Work out the finished part from the listing and answer in its coordinate system (mm). Face numbers are marked on the shaded views. A direction names the side the tool comes from. Coordinates: 2 decimals unless noted, no trailing zeros. Order: outer loops, then holes, each group sorted by start corner. A loop starts at its lowest first (then second) coordinate and runs counter-clockwise, first axis right, second up. Notation, with made-up numbers: M 25,34.25 L 73,34.25 A21 cw 73,56.25 Z; hole C 36.5,-28.75 d3. An arc over 180 degrees is marked long. Use a Markdown table: item, result.
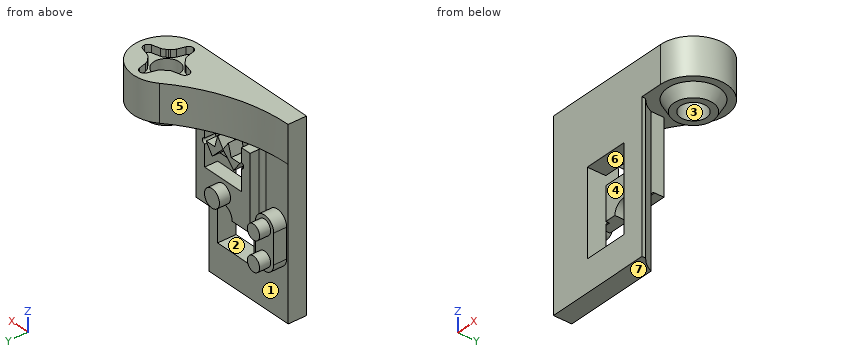
from build123d import *

# Parameters (mm, degrees)
SKETCH2_R           = 9
BOSS_EXTRUDE1_DEPTH = 10
SKETCH3_R           = 7
BOSS_EXTRUDE2_DEPTH = 3
BOSS_EXTRUDE2_TAPER = 30
CUT_EXTRUDE1_DEPTH  = 2
BOSS_EXTRUDE3_DEPTH = 40
SKETCH6_W           = 12
SKETCH6_H           = 23
CUT_EXTRUDE3_DEPTH  = 55.717456081
BOSS_EXTRUDE4_DEPTH = 3.5
SKETCH8_R           = 2
BOSS_EXTRUDE5_DEPTH = 3
SKETCH9_R           = 3.5
CUT_EXTRUDE4_DEPTH  = 52.720402164
BOSS_EXTRUDE6_DEPTH = 3.5
SKETCH11_R          = 2.45
BOSS_EXTRUDE7_DEPTH = 3
BOSS_EXTRUDE9_DEPTH = 3.5
FILLET1_START       = -26.74
FILLET1_DEPTH       = 2.84
FILLET1_START_2     = -11.9
FILLET1_2_DEPTH     = 2.83
FILLET1_START_3     = -21
FILLET1_3_DEPTH     = 21
FILLET1_START_4     = -27.74
FILLET1_4_DEPTH     = 1


with BuildPart() as part:
    # Sketch2 → Boss-Extrude1 (new body)
    with BuildSketch(Plane.XY):
        with BuildLine():
            Line((-35, -9), (0, -9))
            ThreePointArc((0, -9), (-8.437416666, -3.132091953), (-5.872614409, 6.82))
            ThreePointArc((-5.872614409, 6.82), (-19.465199243, -1.204217751), (-35, -4))
            Line((-35, -4), (-35, -9))
        make_face()
        Circle(SKETCH2_R)
    extrude(amount=BOSS_EXTRUDE1_DEPTH)

    # Sketch3 → Boss-Extrude2 (add)
    with BuildSketch(Plane(origin=(0, 0, 0), x_dir=(-1, 0, 0), z_dir=(0, 0, -1))):
        Circle(SKETCH3_R)
    extrude(amount=BOSS_EXTRUDE2_DEPTH, taper=BOSS_EXTRUDE2_TAPER)

    # Sketch4 → Cut-Extrude1 (cut)
    with BuildSketch(Plane.XY.offset(10)):
        with BuildLine():
            Line((1.2, -6.33), (1.8, -4.1378116))
            ThreePointArc((1.8, -4.1378116), (2.058560194, -3.569045514), (2.48, -3.1078116))
            ThreePointArc((2.48, -3.1078116), (2.64989874, -2.964295475), (2.811558399, -2.811558399))
            ThreePointArc((2.811558399, -2.811558399), (2.964295475, -2.64989874), (3.1078116, -2.48))
            ThreePointArc((3.1078116, -2.48), (3.569045514, -2.058560194), (4.1378116, -1.8))
            Line((4.1378116, -1.8), (6.33, -1.2))
            ThreePointArc((6.33, -1.2), (6.992020752, -0.754882576), (7.25, 0))
            ThreePointArc((7.25, 0), (6.992020752, 0.754882576), (6.33, 1.2))
            Line((6.33, 1.2), (4.1378116, 1.8))
            ThreePointArc((4.1378116, 1.8), (3.569045514, 2.058560194), (3.1078116, 2.48))
            ThreePointArc((3.1078116, 2.48), (2.964295475, 2.64989874), (2.811558399, 2.811558399))
            ThreePointArc((2.811558399, 2.811558399), (2.64989874, 2.964295475), (2.48, 3.1078116))
            ThreePointArc((2.48, 3.1078116), (2.058560194, 3.569045514), (1.8, 4.1378116))
            Line((1.8, 4.1378116), (1.2, 6.33))
            ThreePointArc((1.2, 6.33), (0.754882576, 6.992020752), (0, 7.25))
            ThreePointArc((0, 7.25), (-0.754882576, 6.992020752), (-1.2, 6.33))
            Line((-1.2, 6.33), (-1.8, 4.1378116))
            ThreePointArc((-1.8, 4.1378116), (-2.058560194, 3.569045514), (-2.48, 3.1078116))
            ThreePointArc((-2.48, 3.1078116), (-2.64989874, 2.964295475), (-2.811558399, 2.811558399))
            ThreePointArc((-2.811558399, 2.811558399), (-2.964295475, 2.64989874), (-3.1078116, 2.48))
            ThreePointArc((-3.1078116, 2.48), (-3.569045514, 2.058560194), (-4.1378116, 1.8))
            Line((-4.1378116, 1.8), (-6.33, 1.2))
            ThreePointArc((-6.33, 1.2), (-6.992020752, 0.754882576), (-7.25, 0))
            ThreePointArc((-7.25, 0), (-6.992020752, -0.754882576), (-6.33, -1.2))
            Line((-6.33, -1.2), (-4.1378116, -1.8))
            ThreePointArc((-4.1378116, -1.8), (-3.569045514, -2.058560194), (-3.1078116, -2.48))
            ThreePointArc((-3.1078116, -2.48), (-2.964295475, -2.64989874), (-2.811558399, -2.811558399))
            ThreePointArc((-2.811558399, -2.811558399), (-2.64989874, -2.964295475), (-2.48, -3.1078116))
            ThreePointArc((-2.48, -3.1078116), (-2.058560194, -3.569045514), (-1.8, -4.1378116))
            Line((-1.8, -4.1378116), (-1.2, -6.33))
            ThreePointArc((-1.2, -6.33), (-0.754882576, -6.992020752), (0, -7.25))
            ThreePointArc((0, -7.25), (0.754882576, -6.992020752), (1.2, -6.33))
        make_face()
    extrude(amount=-CUT_EXTRUDE1_DEPTH, mode=Mode.SUBTRACT)

    # Sketch5 → Boss-Extrude3 (add)
    with BuildSketch(Plane(origin=(0, 0, 0), x_dir=(-1, 0, 0), z_dir=(0, 0, -1))):
        with BuildLine():
            Line((35, -9), (35, -4))
            Line((35, -4), (9.07, -4))
            ThreePointArc((9.07, -4), (7.791254425, -6.196675271), (6, -8))
            Line((6, -8), (6, -9))
            Line((6, -9), (35, -9))
        make_face()
    extrude(amount=BOSS_EXTRUDE3_DEPTH)

    # Sketch6 → Cut-Extrude3 (cut, through all)
    with BuildSketch(Plane(origin=(0, -4, 0), x_dir=(1, 0, 0), z_dir=(0, 1, 0))):
        with Locations((-17.9, 20)):
            Rectangle(SKETCH6_W, SKETCH6_H)
    extrude(amount=-CUT_EXTRUDE3_DEPTH, mode=Mode.SUBTRACT)

    # Sketch7 → Boss-Extrude4 (add)
    with BuildSketch(Plane(origin=(0, -4, 0), x_dir=(1, 0, 0), z_dir=(0, 1, 0))):
        with BuildLine():
            Line((-34.5, 16), (-34.5, 24))
            ThreePointArc((-34.5, 24), (-31.5, 27), (-28.5, 24))
            Line((-28.5, 24), (-28.5, 16))
            ThreePointArc((-28.5, 16), (-31.5, 13), (-34.5, 16))
        make_face()
    extrude(amount=BOSS_EXTRUDE4_DEPTH)

    # Sketch8 → Boss-Extrude5 (add)
    with BuildSketch(Plane(origin=(0, -0.5, 0), x_dir=(1, 0, 0), z_dir=(0, 1, 0))):
        with Locations(Location((-31.5, 24, 0), (0, 0, 180))):
            Circle(SKETCH8_R)
        with Locations((-31.5, 16)):
            Circle(SKETCH8_R)
    extrude(amount=BOSS_EXTRUDE5_DEPTH)

    # Sketch9 → Cut-Extrude4 (cut, through all)
    with BuildSketch(Plane(origin=(0, 0, -3), x_dir=(-1, 0, 0), z_dir=(0, 0, -1))):
        Circle(SKETCH9_R)
    extrude(amount=-CUT_EXTRUDE4_DEPTH, mode=Mode.SUBTRACT)

    # Sketch10 → Boss-Extrude6 (add)
    with BuildSketch(Plane(origin=(0, -4, 0), x_dir=(1, 0, 0), z_dir=(0, 1, 0))):
        with BuildLine():
            Line((-26.74, 0), (-26.74, 20))
            Line((-26.74, 20), (-20.91, 20))
            ThreePointArc((-20.91, 20), (-17.91, 17), (-14.91, 20))
            Line((-14.91, 20), (-9.07, 20))
            Line((-9.07, 20), (-9.07, 0))
            Line((-9.07, 0), (-11.9, 0))
            Line((-11.9, 0), (-11.9, 3.75))
            ThreePointArc((-11.9, 3.75), (-11.15, 4.5), (-11.9, 5.25))
            Line((-11.9, 5.25), (-11.9, 11))
            Line((-11.9, 11), (-23.9, 11))
            Line((-23.9, 11), (-23.9, 5.25))
            ThreePointArc((-23.9, 5.25), (-24.65, 4.5), (-23.9, 3.75))
            Line((-23.9, 3.75), (-23.9, 0))
            Line((-23.9, 0), (-26.74, 0))
        make_face()
    extrude(amount=BOSS_EXTRUDE6_DEPTH)

    # Sketch11 → Boss-Extrude7 (add)
    with BuildSketch(Plane(origin=(0, -0.5, 0), x_dir=(1, 0, 0), z_dir=(0, 1, 0))):
        with Locations(Location((-17.905833333, 14.5, 0), (0, 0, 180))):
            Circle(SKETCH11_R)
    extrude(amount=BOSS_EXTRUDE7_DEPTH)

    # Sketch12 → Boss-Extrude9 (add)
    with BuildSketch(Plane(origin=(0, -4, 0), x_dir=(1, 0, 0), z_dir=(0, 1, 0))):
        Polygon((-20.58, 4.2), (-19.65, 1), (-17.93, 3.45), (-17.87, 3.45), (-16.15, 1), (-15.22, 4.2), (-12.4, 4.2), (-14.4, 7), (-17.85, 3.55), (-17.95, 3.55), (-21.4, 7), (-23.4, 4.2), align=None)
    extrude(amount=BOSS_EXTRUDE9_DEPTH)

    # Fillet1: read off the stored shape, not the designer's step
    # Fillet1 outline → Fillet1 (add)
    with BuildSketch(Plane.YZ.offset(FILLET1_START)):
        with BuildLine():
            ThreePointArc((-4, -21), (-3.707106781, -20.292893219), (-3, -20))
            Line((-3, -20), (-4, -20))
            Line((-4, -20), (-4, -21))
        make_face()
    extrude(amount=FILLET1_DEPTH)

    # Fillet1 2 outline → Fillet1 2 (add)
    with BuildSketch(Plane.YZ.offset(FILLET1_START_2)):
        with BuildLine():
            ThreePointArc((-4, -21), (-3.707106781, -20.292893219), (-3, -20))
            Line((-3, -20), (-4, -20))
            Line((-4, -20), (-4, -21))
        make_face()
    extrude(amount=FILLET1_2_DEPTH)

    # Fillet1 3 outline → Fillet1 3 (add)
    with BuildSketch(Plane.XY.offset(FILLET1_START_3)):
        with BuildLine():
            Line((-26.74, -4), (-26.74, -3))
            ThreePointArc((-26.74, -3), (-27.032893219, -3.707106781), (-27.74, -4))
            Line((-27.74, -4), (-26.74, -4))
        make_face()
    extrude(amount=FILLET1_3_DEPTH)

    # Fillet1 4 outline → Fillet1 4 (cut)
    with BuildSketch(Plane.YZ.offset(FILLET1_START_4)):
        with BuildLine():
            Line((-2, -19.999999999), (-3, -20))
            ThreePointArc((-3, -20), (-3.707106781, -20.292893219), (-4, -21))
            Line((-4, -21), (-2, -21))
            Line((-2, -21), (-2, -19.999999999))
        make_face()
    extrude(amount=FILLET1_4_DEPTH, mode=Mode.SUBTRACT)


solid = part.part
1. Flat-ended cylindrical pins translate along their axes: P1, Ø5.5, axis at x = -19, z = -13.5, coming from the +Y side; P2, Ø1.5, axis at x = -22, y = 3, coming from the +Z side; P3, Ø3, axis at y = -1.5, z = -7, coming from the -X side; P4, Ø6.5, axis at x = -20.5, z = -3.5, coming from the +Y side. Find the tip coordinate at first contact, or state that the pin passes through.
Answers below:
| item | result |
|---|---|
| P1 | y = 2.5 |
| P2 | through |
| P3 | x = -26.74 |
| P4 | y = -0.5 |
2. Find the intervals of material crossed by probe 1 along Z at (x, y) = (-9.5, 2.5); probe 2 along Z at (x, y) = (-4.5, 1.25); probe 3 along Y at (x, z) = (0, 2), in increasing order.
Answers below:
| item | result |
|---|---|
| probe 1 | 0 to 10 |
| probe 2 | -3 to 8 |
| probe 3 | -9 to -3.5, 3.5 to 9 |
3. Section B-B on z = -32.5 is taken. Determine the outline of the cut face in (x, y), then the cut area to 3 significant figures.
Answers below:
| item | result |
|---|---|
| outline | M -35,-9 L -6,-9 L -6,-8 A10 cw -9.07,-4 L -35,-4 Z |
| area | 138 mm² |
4. For the marked faces 5, 6 and 7, determine the directions among +Z, -Z, +X, -X, +Y, -Y from which every point of the face is accessible in a straight line to the end or side of a thin tool.
Answers below:
| item | result |
|---|---|
| face 5 | +Z, -X, +Y |
| face 6 | +Y, -Y |
| face 7 | -Z, +X, -X, +Y, -Y |
5. For a pull along Y with two mould halves and no side action, classify the marked faces 1, 2, 3 and 4 as +Y half, -Y half, draft (parallel to the pull), parting line (faces both ways), or undercut.
Answers below:
| item | result |
|---|---|
| face 1 | +Y half |
| face 2 | draft |
| face 3 | undercut |
| face 4 | -Y half |
6. Section A-A on x = -22.5 is taken. Determine the outline of the cut face in (y, z).
Answers below:
| item | result |
|---|---|
| outline | M -9,-40 L -4,-40 L -4,-31.5 L -9,-31.5 Z; M -9,-8.5 L -4,-8.5 L -4,-5.46 L -0.5,-5.46 L -0.5,-4.2 L -4,-4.2 L -4,0 L -2.21,0 L -2.21,10 L -9,10 Z; M -4,-20 L -0.5,-20 L -0.5,-11 L -4,-11 Z |
7. Section C-C on x = -8.5 is taken. Determine the outline of the cut face in (y, z), then the cut area to 3 significant figures.
Answers below:
| item | result |
|---|---|
| outline | M -9,-40 L -5.14,-40 L -5.14,0 L 4.72,0 L 4.72,10 L -9,10 Z |
| area | 292 mm² |
